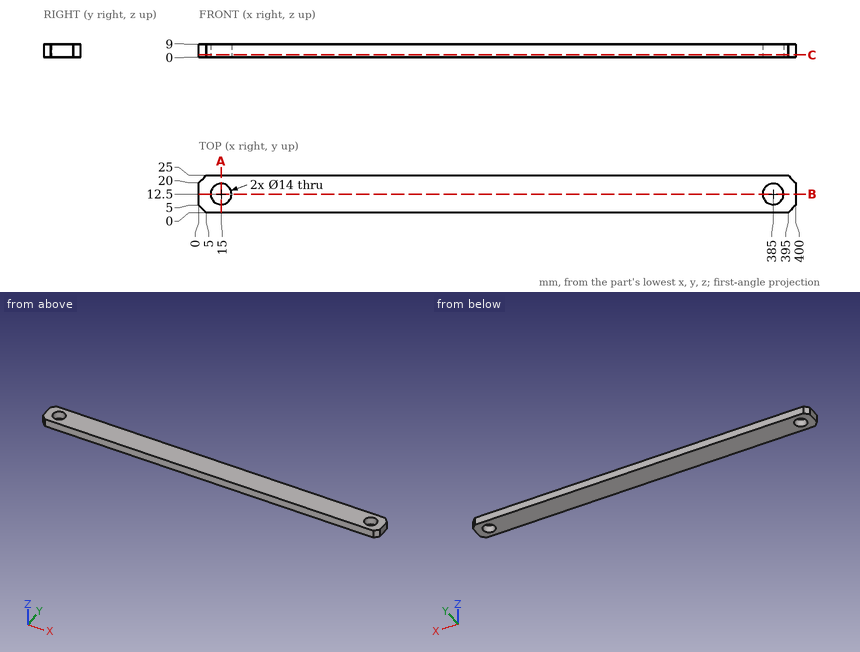
Job drawing, mm, ordinate dimensions from the low corner. One solid piece. Coordinates: 2 decimals unless noted, no trailing zeros. Write each loop counter-clockwise with the first axis right and the second up, starting at its lowest first coordinate (ties: lowest second). Pieces come first, ordered by that corner, then holes. Notation, with made-up numbers: (38.25, 8.25) - (92.25, 8.25) arc R21 ccw to (92.25, 26.25) - close; hole circle Ø10 at (26, 54). An arc over 180 degrees is marked (long way). Use a Markdown table: item, result. Add a question column.
Item 1: Drill centre lines: L1, parallel to Y at x = 15, z = 6.75; L2, parallel to X at y = 16.75, z = 4; L3, parallel to X at y = 8, z = 4.5. Where is each one in solid material? Low to high. Write a range as from..to.
Item 2: Band-saw the part on B-B, the plane y = 12.5. Give the cut face in (x, z), and give its area (3 significant figures).
Item 3: Band-saw the part on C-C, the plane z = 1.75. Give the cut face in (x, y).
Item 4: Band-saw the part on A-A, the plane x = 15. Give the cut face in (y, z).
Numbers:
| question | item | result |
|---|---|---|
| 1 | L1 | 0..5.5, 19.5..25 |
| 1 | L2 | 0..9.44, 20.56..379.44, 390.56..400 |
| 1 | L3 | 0..9.64, 20.36..379.64, 390.36..400 |
| 2 | outline | (0, 0) - (8, 0) - (8, 9) - (0, 9) - close; (22, 0) - (378, 0) - (378, 9) - (22, 9) - close; (392, 0) - (400, 0) - (400, 9) - (392, 9) - close |
| 2 | area | 3,350 mm2 |
| 3 | outline | (0, 5) - (5, 0) - (395, 0) - (400, 5) - (400, 20) - (395, 25) - (5, 25) - (0, 20) - close; hole circle Ø14 at (15, 12.5); hole circle Ø14 at (385, 12.5) |
| 4 | outline | (0, 0) - (5.5, 0) - (5.5, 9) - (0, 9) - close; (19.5, 0) - (25, 0) - (25, 9) - (19.5, 9) - close |
